The listing builds one solid part. Answer for the finished solid, in the listing's coordinates (mm). Face numbers are marked on the shaded views. Give positions to 0.01 mm unless a question says otherwise; leave off trailing zeros. Order: outer loops, then holes, each group sorted by start corner. A loop starts at its lowest first (then second) coordinate and runs counter-clockwise, first axis right, second up. Notation, with made-up numbers: (-28.75, 75.25) - (29.25, 75.25) arc R32 ccw to (29.25, 113.25) - close; hole circle Ø5 at (-26.5, 6). An arc over 180 degrees is marked (long way). Use a Markdown table: item, result. Add a question column.
1) Flat-ended cylindrical pins translate along their axes: pin 1 (1.5 mm diameter, centred on y = 14, z = 8, fed in from +X); pin 2 (4 mm diameter, centred on x = 0, z = -12.7, fed in from -Y); pin 3 (4 mm diameter, centred on x = 1, z = 13, fed in from +Y); pin 4 (3 mm diameter, centred on x = 0, z = 12.7, fed in from +Y). Find the tip coordinate at first contact, or state that the pin passes through.
2) Find section A-A, the plane y = 8. Determine the outline of the cut face in (x, z), plus the area to 3 significant figures.
3) Find section D-D, the plane x = 3. Determine the outline of the cut face in (y, z), plus the area to 3 significant figures.
4) The mould has two halves that part along Y. Classify the marked faces 1, 2 and 3: released by +Y, released by -Y, zero draft, split by the parting line, or undercut.
5) Straight lines are drawn through the part: line 1 (X direction, y = 2, z = -2); line 2 (Y direction, x = 1, z = 7). For each, find the intervals that lie inside material, in ascending order.
6) Find section B-B, the plane z = 12. Determine the outline of the cut face in (x, y).
7) Find section C-C, the plane z = 2.5. Determine the outline of the cut face in (x, y).
from build123d import *

# Parameters (mm, degrees)
F0_W     = 12.7
F0_H     = 38.1
F1_DEPTH = 1.5875
F2_W     = 1.5875
F2_H     = 38.1
F3_DEPTH = 25.4
F4_R     = 6.35
F5_R     = 1.5875
F6_DEPTH = 1.5875
F8_DEPTH = 1.5875


with BuildPart() as f1:
    # F0 (on Front) → F1 (new body)
    with BuildSketch(Plane.XZ):
        Rectangle(F0_W, F0_H)
    extrude(amount=F1_DEPTH)

    # F2 (on face) → F3 (join)
    with BuildSketch(Plane.XZ.offset(1.5875)):
        with Locations((-5.55625, 0)):
            Rectangle(F2_W, F2_H)
    extrude(amount=-F3_DEPTH)

    # F4
    f4_edges = [f1.edges().sort_by_distance(p)[0] for p in [
        (6.35, -0.79375, 19.05),
        (-5.55625, 23.8125, 19.05),
        (6.35, -0.79375, -19.05),
        (-5.55625, 23.8125, -19.05),
    ]]
    fillet(f4_edges, radius=F4_R)

    # F5 (on face) → F6 (cut, through all)
    with BuildSketch(Plane.XZ.offset(1.5875)):
        with Locations((0, 12.7)):
            Circle(F5_R)
        with Locations((0, -12.7)):
            Circle(F5_R)
    extrude(amount=-F6_DEPTH, mode=Mode.SUBTRACT)

    # F7 (on face) → F8 (cut, through all)
    with BuildSketch(Plane.YZ.offset(-4.7625)):
        with BuildLine():
            ThreePointArc((7.9375, 12.7), (7.4725320151, 13.8225320151), (6.35, 14.2875))
            Line((6.35, 14.2875), (6.35, 11.1125))
            ThreePointArc((6.35, 11.1125), (7.4725320151, 11.5774679849), (7.9375, 12.7))
        make_face()
        with BuildLine():
            Line((15.875, 14.2875), (6.35, 14.2875))
            ThreePointArc((6.35, 14.2875), (7.4725320151, 13.8225320151), (7.9375, 12.7))
            ThreePointArc((7.9375, 12.7), (7.4725320151, 11.5774679849), (6.35, 11.1125))
            Line((6.35, 11.1125), (15.875, 11.1125))
            ThreePointArc((15.875, 11.1125), (14.2875, 12.7), (15.875, 14.2875))
        make_face()
        with BuildLine():
            Line((6.35, 11.1125), (6.35, 14.2875))
            ThreePointArc((6.35, 14.2875), (4.7625, 12.7), (6.35, 11.1125))
        make_face()
        with BuildLine():
            ThreePointArc((17.4625, 12.7), (16.9975320151, 13.8225320151), (15.875, 14.2875))
            Line((15.875, 14.2875), (15.875, 11.1125))
            ThreePointArc((15.875, 11.1125), (16.9975320151, 11.5774679849), (17.4625, 12.7))
        make_face()
        with BuildLine():
            Line((15.875, 11.1125), (15.875, 14.2875))
            ThreePointArc((15.875, 14.2875), (14.2875, 12.7), (15.875, 11.1125))
        make_face()
        with BuildLine():
            ThreePointArc((7.9375, -12.7), (7.4725320151, -11.5774679849), (6.35, -11.1125))
            Line((6.35, -11.1125), (6.35, -14.2875))
            ThreePointArc((6.35, -14.2875), (7.4725320151, -13.8225320151), (7.9375, -12.7))
        make_face()
        with BuildLine():
            Line((15.875, -11.1125), (6.35, -11.1125))
            ThreePointArc((6.35, -11.1125), (7.4725320151, -11.5774679849), (7.9375, -12.7))
            ThreePointArc((7.9375, -12.7), (7.4725320151, -13.8225320151), (6.35, -14.2875))
            Line((6.35, -14.2875), (15.875, -14.2875))
            ThreePointArc((15.875, -14.2875), (14.2875, -12.7), (15.875, -11.1125))
        make_face()
        with BuildLine():
            Line((6.35, -14.2875), (6.35, -11.1125))
            ThreePointArc((6.35, -11.1125), (4.7625, -12.7), (6.35, -14.2875))
        make_face()
        with BuildLine():
            ThreePointArc((17.4625, -12.7), (16.9975320151, -11.5774679849), (15.875, -11.1125))
            Line((15.875, -11.1125), (15.875, -14.2875))
            ThreePointArc((15.875, -14.2875), (16.9975320151, -13.8225320151), (17.4625, -12.7))
        make_face()
        with BuildLine():
            Line((15.875, -14.2875), (15.875, -11.1125))
            ThreePointArc((15.875, -11.1125), (14.2875, -12.7), (15.875, -14.2875))
        make_face()
    extrude(amount=-F8_DEPTH, mode=Mode.SUBTRACT)


solid = f1.part
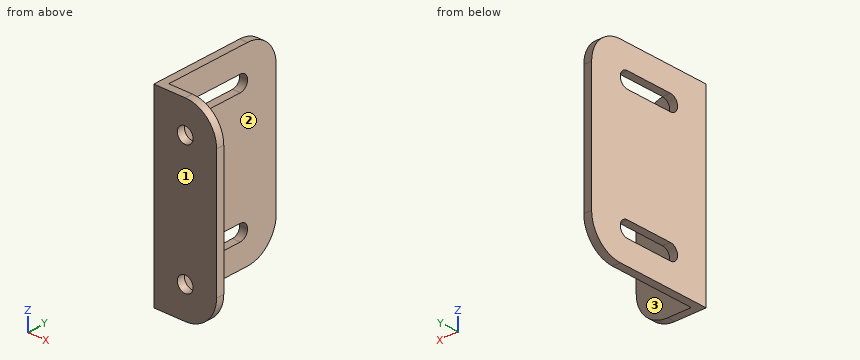
The answers:
| question | item | result |
|---|---|---|
| 1 | pin 1 | x = -4.76 |
| 1 | pin 2 | y = -1.59 |
| 1 | pin 3 | y = 0 |
| 1 | pin 4 | through |
| 2 | outline | (-6.35, -19.05) - (-4.76, -19.05) - (-4.76, -14.29) - (-6.35, -14.29) - close; (-6.35, -11.11) - (-4.76, -11.11) - (-4.76, 11.11) - (-6.35, 11.11) - close; (-6.35, 14.29) - (-4.76, 14.29) - (-4.76, 19.05) - (-6.35, 19.05) - close |
| 2 | area | 50.4 mm2 |
| 3 | outline | (-1.59, -18.3) - (0, -18.3) - (0, 18.3) - (-1.59, 18.3) - close |
| 3 | area | 58.1 mm2 |
| 4 | face 1 | released by -Y |
| 4 | face 2 | zero draft |
| 4 | face 3 | released by +Y |
| 5 | line 1 | -6.35 to -4.76 |
| 5 | line 2 | -1.59 to 0 |
| 6 | outline | (-6.35, -1.59) - (-1.42, -1.59) - (-1.42, 0) - (-4.76, 0) - (-4.76, 4.93) - (-6.35, 4.93) - close; (-6.35, 17.3) - (-4.76, 17.3) - (-4.76, 23.81) - (-6.35, 23.81) - close; (1.42, -1.59) - (6.35, -1.59) - (6.35, 0) - (1.42, 0) - close |
| 7 | outline | (-6.35, -1.59) - (6.35, -1.59) - (6.35, 0) - (-4.76, 0) - (-4.76, 23.81) - (-6.35, 23.81) - close |
